```python
from build123d import *

# Parameters (mm, degrees)
SKETCH1_R           = 21
BOSS_EXTRUDE1_DEPTH = 10
SKETCH2_R           = 15
CUT_EXTRUDE1_DEPTH  = 4
SKETCH3_R           = 19
SKETCH3_R_2         = 5
CUT_EXTRUDE2_DEPTH  = 4
SKETCH4_R           = 2
CUT_EXTRUDE3_DEPTH  = 32.336879232
SKETCH5_R           = 2
CUT_EXTRUDE4_DEPTH  = 31.298514815


with BuildPart() as part:
    # Sketch1 → Boss-Extrude1 (new body)
    with BuildSketch(Plane(origin=(0, 0, 0), x_dir=(1, 0, 0), z_dir=(0, 1, 0))):
        with Locations(Location((0, 0, 0), (0, 0, 270))):
            Circle(SKETCH1_R)
    extrude(amount=BOSS_EXTRUDE1_DEPTH)

    # Sketch2 → Cut-Extrude1 (cut)
    with BuildSketch(Plane(origin=(0, 10, 0), x_dir=(1, 0, 0), z_dir=(0, 1, 0))):
        with Locations(Location((0, 0, 0), (0, 0, 270))):
            Circle(SKETCH2_R)
    extrude(amount=-CUT_EXTRUDE1_DEPTH, mode=Mode.SUBTRACT)

    # Sketch3 → Cut-Extrude2 (cut)
    with BuildSketch(Plane.XZ):
        with Locations(Location((0, 0, 0), (0, 0, 270))):
            Circle(SKETCH3_R)
        with Locations(Location((0, 0, 0), (0, 0, 270))):
            Circle(SKETCH3_R_2, mode=Mode.SUBTRACT)
    extrude(amount=-CUT_EXTRUDE2_DEPTH, mode=Mode.SUBTRACT)

    # Sketch4 → Cut-Extrude3 (cut, through all)
    with BuildSketch(Plane.XZ):
        with Locations(Location((0, 0, 0), (0, 0, 270))):
            Circle(SKETCH4_R)
    extrude(amount=-CUT_EXTRUDE3_DEPTH, mode=Mode.SUBTRACT)

    # Sketch5 → Cut-Extrude4 (cut, through all)
    with BuildSketch(Plane.XZ.offset(-4)):
        with Locations(Location((0, 12, 0), (0, 0, 270))):
            Circle(SKETCH5_R)
        with Locations(Location((10.392304845, 6, 0), (0, 0, 270))):
            Circle(SKETCH5_R)
        with Locations(Location((10.392304845, -6, 0), (0, 0, 270))):
            Circle(SKETCH5_R)
        with Locations(Location((0, -12, 0), (0, 0, 270))):
            Circle(SKETCH5_R)
        with Locations(Location((-10.392304845, -6, 0), (0, 0, 270))):
            Circle(SKETCH5_R)
        with Locations(Location((-10.392304845, 6, 0), (0, 0, 270))):
            Circle(SKETCH5_R)
    extrude(amount=-CUT_EXTRUDE4_DEPTH, mode=Mode.SUBTRACT)


solid = part.part
```
Work out the finished part from the listing and answer in its coordinate system (mm). A direction names the side the tool comes from. Coordinates: 2 decimals unless noted, no trailing zeros. Loops run counter-clockwise (first coordinate to the right, second up) from the corner with the lowest first, then second, coordinate; pieces in that order, holes last. Notation, with made-up numbers: M 37,71 L 53,71 A10 ccw 53,77 Z; hole C -11,88.5 d3. An arc over 180 degrees is marked long. Use CSV: the item, a comma, the result in double quotes. Start each with the question number.
(1) Given pin 1 Ø4 at (x, y) = (-14, 7) entering from +Z; pin 2 Ø4.5 at (x, z) = (0, -12) entering from +Y; pin 3 Ø2 at (x, y) = (9.5, 1.5) entering from -Z, each flat-ended and moving along its own axis, determine where each tip first touches the part or whether it passes through.
(2) Find section C-C, the plane y = 1.75. Give the vertices of the cut face in (x, z).
(3) For faces 1 (the face through (-1.2, 5, -10.4)), 2 (the face through (-4, 4, -4)), 3 (the face through (0, 6, 3)), determine the directions among +Z, -Z, +X, -X, +Y, -Y from which every point of the face is accessible in a straight line to the end or side of a thin tool.
(4) Consider line 1 (X direction, y = 2, z = 0); line 2 (Y direction, x = -1, z = 5); line 3 (Y direction, x = -3.5, z = 18). Determine where each line is inside the solid, lowest interval first.
(5) Find section D-D, the plane z = -6. Give the vertices of the cut face in (x, y).
(6) Find section B-B, the plane z = 0. Give the vertices of the cut face in (x, y).
(7) Find section A-A, the plane x = 0. Give the vertices of the cut face in (y, z).
Recorded:
1,pin 1,"stops at z = 17.23"
1,pin 2,"stops at y = 6"
1,pin 3,"stops at z = -19.2"
2,outline,"C 0,0 d42; C 0,0 d10; hole C 0,0 d38; hole C 0,0 d4"
3,face 1,"+Y, -Y"
3,face 2,"-Y"
3,face 3,"+Y"
4,line 1,"x = -21 to -19, -5 to -2, 2 to 5, 19 to 21"
4,line 2,"y = 4 to 6"
4,line 3,"y = 4 to 10"
5,outline,"M -20.12,0 L -18.03,0 L -18.03,4 L -12.39,4 L -12.39,6 L -13.75,6 L -13.75,10 L -20.12,10 Z; M -8.39,4 L 8.39,4 L 8.39,6 L -8.39,6 Z; M 12.39,4 L 18.03,4 L 18.03,0 L 20.12,0 L 20.12,10 L 13.75,10 L 13.75,6 L 12.39,6 Z"
6,outline,"M -21,0 L -19,0 L -19,4 L -5,4 L -5,0 L -2,0 L -2,6 L -15,6 L -15,10 L -21,10 Z; M 2,0 L 5,0 L 5,4 L 19,4 L 19,0 L 21,0 L 21,10 L 15,10 L 15,6 L 2,6 Z"
7,outline,"M 0,-21 L 10,-21 L 10,-15 L 6,-15 L 6,-14 L 4,-14 L 4,-19 L 0,-19 Z; M 0,-5 L 4,-5 L 4,-10 L 6,-10 L 6,-2 L 0,-2 Z; M 0,2 L 6,2 L 6,10 L 4,10 L 4,5 L 0,5 Z; M 0,19 L 4,19 L 4,14 L 6,14 L 6,15 L 10,15 L 10,21 L 0,21 Z"
